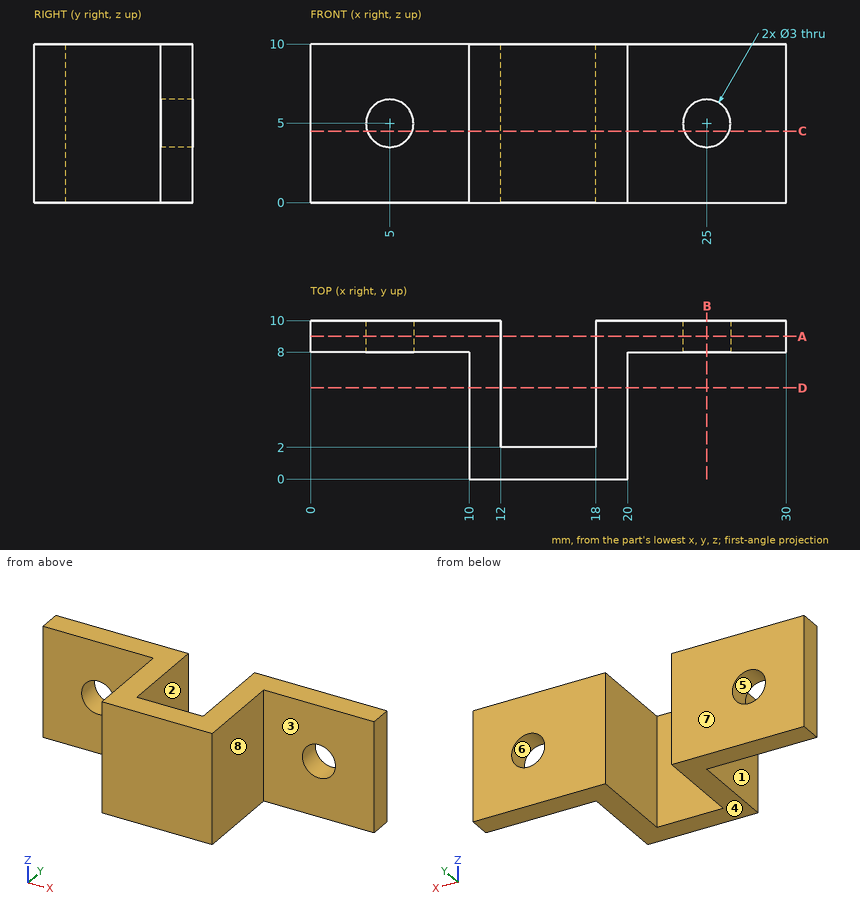
Geometry check sheet. Reference: drawing and pictorial views, mm from the part's lowest x, y, z. A direction names the side the tool comes from. Give positions to 0.01 mm unless a question says otherwise; leave off trailing zeros. Order: outer loops, then holes, each group sorted by start corner. A loop starts at its lowest first (then second) coordinate and runs counter-clockwise, first axis right, second up. Notation, with made-up numbers: M -22.75,-33 L 36.25,-33 A9 cw 36.25,-25 Z; hole C -39.75,-11.75 d8. An arc over 180 degrees is marked long. Answer as a JSON object with one key per item and string values. Group by question number.
1) Mould release check, pull along X, two halves, no side actions. Record for the marked faces 5, 6, 7 and 8: released by +X, released by -X, zero draft, split by the parting line, or undercut.
2) Access from +Z, -Z, +X, -X, +Y, -Y to the whole of each face (thin tool, end or side, straight path). Record for the marked faces 1, 2, 3 and 4.
3) Cross-section at C-C (z = 4.5). Enter the section's corners in (x, y).
4) Cross-section at D-D (y = 5.75). Enter the section's corners in (x, z), then the cut area to 3 significant figures.
5) Cross-section at B-B (x = 25). Enter the section's corners in (y, z), then the cut area to 3 significant figures.
6) Depth check by flat-ended pin: pin 1 Ø2 at (y, z) = (1.5, 3.5) entering from -X; pin 2 Ø3 at (x, z) = (4, 5.5) entering from -Y. Enter the tip coordinate at first touch or a pass-through.
7) Scan lines: line 1 along X through (y, z) = (8.85, 5); line 2 along Z through (x, y) = (5, 9.5); line 3 along X through (y, z) = (5.75, 8.75). Record each from-to range of solid material in increasing order. Write a range as [from, to].
8) Cross-section at A-A (y = 9). Enter the section's corners in (x, z), then the cut area to 3 significant figures.
Result sheet:
{
 "1": {"face 5": "undercut", "face 6": "undercut", "face 7": "zero draft", "face 8": "released by +X"},
 "2": {"face 1": "+Z, -Z, -X, -Y", "face 2": "+Z, -Z, +Y", "face 3": "+Z, -Z, +X, -Y", "face 4": "-Z, +X, -X, +Y, -Y"},
 "3": {"outline": "M 0,8 L 3.59,8 L 3.59,10 L 0,10 Z; M 6.41,8 L 10,8 L 10,0 L 20,0 L 20,8 L 23.59,8 L 23.59,10 L 18,10 L 18,2 L 12,2 L 12,10 L 6.41,10 Z; M 26.41,8 L 30,8 L 30,10 L 26.41,10 Z"},
 "4": {"outline": "M 10,0 L 12,0 L 12,10 L 10,10 Z; M 18,0 L 20,0 L 20,10 L 18,10 Z", "area": "40.0 mm2"},
 "5": {"outline": "M 8,0 L 10,0 L 10,3.5 L 8,3.5 Z; M 8,6.5 L 10,6.5 L 10,10 L 8,10 Z", "area": "14.0 mm2"},
 "6": {"pin 1": "stops at x = 10", "pin 2": "stops at y = 8"},
 "7": {"line 1": "x = [0, 3.5], [6.5, 12], [18, 23.5], [26.5, 30]", "line 2": "z = [0, 3.5], [6.5, 10]", "line 3": "x = [10, 12], [18, 20]"},
 "8": {"outline": "M 0,0 L 12,0 L 12,10 L 0,10 Z; M 18,0 L 30,0 L 30,10 L 18,10 Z; hole C 5,5 d3; hole C 25,5 d3", "area": "226 mm2"}
}
